Autodesk Inventor part; units mm, degrees
ref_plane "YZ Plane" through (0, 0, 0) normal (1, 0, 0) x (0, 1, 0)
ref_plane "XZ Plane" through (0, 0, 0) normal (0, 1, 0) x (-1, 0, 0)
ref_plane "XY Plane" through (0, 0, 0) normal (0, 0, 1) x (1, 0, 0)
sketch "草图1" plane through (0, 0, 0) normal (0, 0, 1) x (1, 0, 0)
  circle A0 centre (0, 0) radius 100
  line L0 (-25, -96.8246) -> (25, -96.8246)
  line L1 (25, -96.8246) -> (25, -118)
  line L2 (25, -118) -> (-25, -118)
  line L3 (-25, -118) -> (-25, -96.8246)
  line L4 (0, -100) -> (-25, -100)
  arc A1 (28, -99.1211) -> (102.0345, 14.0701) centre (0, 0) ccw
  line L5 (25, -118) -> (28, -118)
  line L6 (28, -118) -> (28, -99.1211)
  line L7 (98.9752, 14.2797) -> (107.1784, 43.1364)
  line L8 (107.1784, 43.1364) -> (110.0641, 42.3161)
  line L9 (110.0641, 42.3161) -> (102.0345, 14.0701)
  line L10 (-25, 96.8246) -> (-25, 300)
  line L11 (-25, 300) -> (175, 300)
  line L12 (175, 300) -> (96.8246, 25)
  dimension "d0" = 200
  dimension "d1" = 50
  dimension "d2" = 18
  dimension "d3" = 3
  dimension "d4" = 3
  dimension "d5" = 3
  dimension "d6" = 200
  dimension "d7" = 25
  dimension "d8" = 25
  dimension "d9" = 5
  dimension "d10" = 300
  dimension "d11" = 30
extrude "拉伸1" add sketch "草图1" against normal blind 398 contours A0 L7 L8 L9 A1 L6 L5 L1
sketch "草图2" plane through (28, -118, 0) normal (1, 0, 0) x (0, 0, -1)
  circle A0 centre (293, 10) radius 2.5
  circle A1 centre (345, 10) radius 2.5
  line L0 (0, 0) -> (398, 0)
  line L1 (398, 18.8789) -> (398, 0)
  point P0 (0, 118)
  dimension "d14" = 5
  dimension "d15" = 5
  dimension "d16" = 10
  dimension "d17" = 10
  dimension "d18" = 53
  dimension "d19" = 105
extrude "拉伸2" cut sketch "草图2" against normal blind 3
pattern_linear "矩形阵列1" count 3 spacing 120 along (0, 0, 1) of "拉伸2"
sketch "草图3" plane through (102.0345, 14.0701, 0) normal (0.9619, -0.2734, 0) x (0, 0, -1)
  circle A0 centre (390, 14.3651) radius 2.5
  circle A1 centre (368, 14.3651) radius 2.5
  line L0 (0, 29.3651) -> (398, 29.3651)
  line L1 (398, 29.3651) -> (398, 0)
  point P0 (0, -41.4342)
  dimension "d25" = 5
  dimension "d26" = 5
  dimension "d27" = 15
  dimension "d28" = 15
  dimension "d29" = 8
  dimension "d30" = 30
extrude "拉伸3" cut sketch "草图3" against normal blind 3
pattern_linear "矩形阵列2" count 4 spacing 120 along (0, 0, 1) of "拉伸3"
properties part number "装填斗后罩"
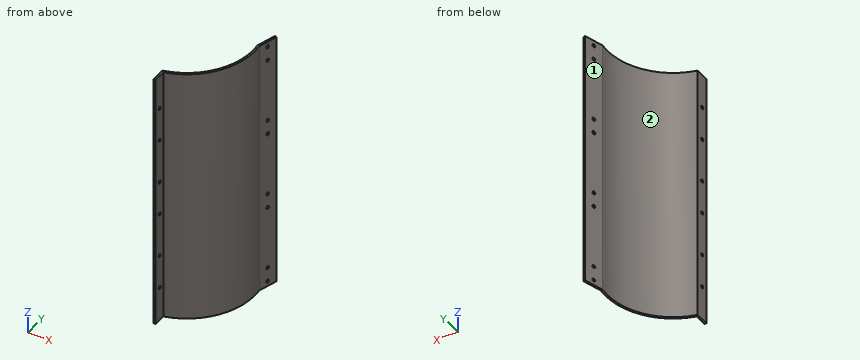
Build history of the part. All positions in model axes, mm. Face numbers are marked on the shaded views. Give positions to 0.01 mm unless a question says otherwise; leave off trailing zeros. Order: outer loops, then holes, each group sorted by start corner. A loop starts at its lowest first (then second) coordinate and runs counter-clockwise, first axis right, second up. Notation, with made-up numbers: M 83.25,25 L 127.25,25 A14 ccw 127.25,34 Z; hole C 47,23 d2. An arc over 180 degrees is marked long. Write item = value, one per line. Start each with the question number.
(1) Slice it at C-C on y = -65. Write the cut outline in (x, z).
(2) Probe L1, parallel to X at y = -101, z = -380; L2, parallel to Y at x = 26.2, z = -105; L3, parallel to Y at x = 25.85, z = -53. List the from-to ranges inside material, lowest first. Write a range as [from, to].
(3) Pin check, flat tips, straight feed: pin 1 Ø5 at (x, z) = (85, -133.5) entering from -Y; pin 2 Ø5 at (y, z) = (-30.5, -190) entering from -X; pin 3 Ø8 at (y, z) = (-108, -105) entering from -X; pin 4 Ø6 at (y, z) = (3.5, -212.5) entering from -X. Stop position of each tip, or through.
(4) Slice it at A-A on z = -258. Write the cut outline in (x, y), plus the area to 3 significant figures.
(5) Slice it at B-B on x = 80. Write the cut outline in (y, z), plus the area to 3 significant figures.
(6) Two-plate mould, pull along Y, no slides. Class the marked faces 1 and 2: released by +Y, released by -Y, zero draft, split by the parting line, or undercut.
Responses:
q1.outline = M 75.99,-398 L 79.9,-398 L 79.9,0 L 75.99,0 Z
q2.L1 = [25, 28]
q2.L2 = [-118, -110.5], [-105.5, -96.51]
q2.L3 = [-118, -110.5], [-105.5, -96.6]
q3.pin_1 = -61.67
q3.pin_2 = 94.4
q3.pin_3 = 25
q3.pin_4 = 99.79
q4.outline = M 25,-118 L 28,-118 L 28,-99.12 A103 ccw 102.03,14.07 L 110.06,42.32 L 107.18,43.14 L 98.98,14.28 A100 cw 25,-96.82 Z
q4.area = 590 mm2
q5.outline = M -64.88,-398 L -60,-398 L -60,0 L -64.88,0 Z
q5.area = 1,940 mm2
q6.face_1 = released by +Y
q6.face_2 = undercut
